```python
from build123d import *

# Parameters (mm, degrees)
SCHIZZO1_R                   = 1.75
ESTRUSIONE_ESTRUSIONE1_DEPTH = 3
ESTRUSIONE_ESTRUSIONE2_START = 11
SCHIZZO2_R                   = 1.4
ESTRUSIONE_ESTRUSIONE2_DEPTH = 4
TAGLIO_ESTRUSIONE1_DEPTH     = 53.736941512
SCHIZZO4_R                   = 1.75
TAGLIO_ESTRUSIONE2_DEPTH     = 53.736941512


with BuildPart() as part:
    # Schizzo1 → Estrusione-Estrusione1 (new body)
    with BuildSketch(Plane(origin=(0, 0, 0), x_dir=(1, 0, 0), z_dir=(0, 1, 0))):
        with BuildLine():
            Line((-46.5, -4.15), (46.5, -4.15))
            ThreePointArc((46.5, -4.15), (50.65, 0), (46.5, 4.15))
            Line((46.5, 4.15), (-46.5, 4.15))
            ThreePointArc((-46.5, 4.15), (-50.65, 0), (-46.5, -4.15))
        make_face()
        with Locations(Location((46.5, 0, 0), (0, 0, 270))):
            Circle(SCHIZZO1_R, mode=Mode.SUBTRACT)
        with Locations(Location((-46.5, 0, 0), (0, 0, 270))):
            Circle(SCHIZZO1_R, mode=Mode.SUBTRACT)
    extrude(amount=ESTRUSIONE_ESTRUSIONE1_DEPTH)

    # Schizzo2 → Estrusione-Estrusione2 (add)
    with BuildSketch(Plane(origin=(0, 0, 0), x_dir=(0, 0, -1), z_dir=(1, 0, 0)).offset(ESTRUSIONE_ESTRUSIONE2_START)):
        with BuildLine():
            Line((10.15, 7.6), (4.15, 7.6))
            Line((4.15, 7.6), (0, 3))
            Line((0, 3), (4.15, 3))
            Line((4.15, 3), (4.15, 0))
            Line((4.15, 0), (10.15, 0))
            ThreePointArc((10.15, 0), (13.95, 3.8), (10.15, 7.6))
        make_face()
        with Locations((10.15, 3.8)):
            Circle(SCHIZZO2_R, mode=Mode.SUBTRACT)
    estrusione_estrusione2 = extrude(amount=-ESTRUSIONE_ESTRUSIONE2_DEPTH)

    # Specchia1: Estrusione-Estrusione2 across plane
    add(estrusione_estrusione2.mirror(Plane(origin=(0, 0, 0), x_dir=(0, 0, 1), z_dir=(1, 0, 0))))

    # Schizzo3 → Taglio-Estrusione1 (cut, through all)
    with BuildSketch(Plane(origin=(0, 3, 0), x_dir=(1, 0, 0), z_dir=(0, 1, 0))):
        Polygon((-25, -4.15), (-20, -1.15), (20, -1.15), (25, -4.15), align=None)
    extrude(amount=-TAGLIO_ESTRUSIONE1_DEPTH, mode=Mode.SUBTRACT)

    # Schizzo4 → Taglio-Estrusione2 (cut, through all)
    with BuildSketch(Plane(origin=(0, 3, 0), x_dir=(1, 0, 0), z_dir=(0, 1, 0))):
        with Locations(Location((0, 1.5, 0), (0, 0, 270))):
            Circle(SCHIZZO4_R)
    extrude(amount=-TAGLIO_ESTRUSIONE2_DEPTH, mode=Mode.SUBTRACT)


solid = part.part
```
Can you work these out from the model? Positions are in its coordinate system, mm. A direction names the side the tool comes from. Round coordinates to 2 decimals unless told otherwise and drop trailing zeros. Order: outer loops, then holes, each group sorted by start corner. A loop starts at its lowest first (then second) coordinate and runs counter-clockwise, first axis right, second up.
(1) If we section it at C-C (x = 26): Please give me the cut outline in (y, z).
Results are:
outline: (0, -4.15) - (3, -4.15) - (3, 4.15) - (0, 4.15) - close
(2) On a 3-axis mill with a long thin cutter (end or side, diameter ignored), from which of +Z, -Z, +X, -X, +Y, -Y can I reach the whole of each face in a straight line? I mean faces 1 (the face through (29, 1, -4.15)), 2 (the face through (0, 1, -4.15)), 3 (the face through (22.465, 1.521, 2.629)). Say none if no direction works.
Results are:
face 1: -Z, +X, +Y, -Y
face 2: -Z, +Y, -Y
face 3: +Z, +Y, -Y
(3) If I drill on L1, parallel to X at y = 2, z = -8.5; L2, parallel to X at y = 1.55, z = 0; L3, parallel to Y at x = -24.5, z = -3.25, over which ranges is the centre line in solid material (lowest first)?
Results are:
L1: x = -11 to -7, 7 to 11
L2: x = -50.65 to -48.25, -44.75 to -0.9, 0.9 to 44.75, 48.25 to 50.65
L3: y = 0 to 3
(4) If we section it at B-B (y = 6.25): Please give me the cut outline in (x, z), plus the area to 3 significant figures.
Results are:
outline: (-11, -13.05) - (-7, -13.05) - (-7, -2.93) - (-11, -2.93) - close; (7, -13.05) - (11, -13.05) - (11, -2.93) - (7, -2.93) - close
area: 81.0 mm2
(5) We'd pull the mould along Z, two halves only. Please class faces 4 (the face through (-48.21, 1.48, -0.38)), 5 (the face through (50.65, 1.48, 0.09)), 6 (the face through (-22.535, 1.521, 2.671)), 7 (the face through (11, 4, -8)): +Z half, -Z half, draft (parallel to the pull), parting line (faces both ways), or undercut.
Results are:
face 4: undercut
face 5: parting line
face 6: +Z half
face 7: draft
(6) I'm going to push flat-ended pins straight in: pin 1 (5 mm diameter, centred on x = 3.5, z = 1.5, fed in from -Y); pin 2 (4.5 mm diameter, centred on x = -46.5, z = 0, fed in from +Y); pin 3 (2.5 mm diameter, centred on y = 5, z = -4, fed in from -X); pin 4 (3 mm diameter, centred on x = 10.5, z = -1.5, fed in from +Y). Where does each tip first touch, or does it pass through?
Results are:
pin 1: stops at y = 0
pin 2: stops at y = 3
pin 3: stops at x = -11
pin 4: stops at y = 6.33
(7) If we section it at A-A (z = -6): Please give me the cut outline in (x, y), plus the area to 3 significant figures.
Results are:
outline: (-11, 0) - (-7, 0) - (-7, 7.6) - (-11, 7.6) - close; (7, 0) - (11, 0) - (11, 7.6) - (7, 7.6) - close
area: 60.8 mm2
